Autodesk Inventor part; units mm, degrees
ref_plane "YZ Plane" through (0, 0, 0) normal (1, 0, 0) x (0, 1, 0)
ref_plane "XZ Plane" through (0, 0, 0) normal (0, 1, 0) x (-1, 0, 0)
ref_plane "XY Plane" through (0, 0, 0) normal (0, 0, 1) x (1, 0, 0)
sketch "Sketch1" plane through (0, 0, 0) normal (0, 1, 0) x (-1, 0, 0)
  line L0 (-1.27, 1.27) -> (1.27, 1.27)
  line L1 (1.27, 1.27) -> (1.27, -1.27)
  line L2 (1.27, -1.27) -> (-1.27, -1.27)
  line L3 (-1.27, -1.27) -> (-1.27, 1.27)
  line L4 (-1.27, 1.27) -> (1.27, -1.27) construction
  line L5 (1.27, 1.27) -> (-1.27, -1.27) construction
  point P0 (0, 0)
  dimension "d0" = 2.54
  dimension "d1" = 2.54
extrude "Extrusion1" add sketch "Sketch1" along normal blind 10
sketch "Sketch2" plane through (0, 10, 0) normal (0, 1, 0) x (1, 0, 0)
  circle A0 centre (0, 0) radius 0.375
  dimension "d4" = 0.75
extrude "Extrusion2" cut sketch "Sketch2" against normal blind 100
fillet "Fillet1" radius 0.5 4 edges at (-1.27, 5, 1.27) (1.27, 5, 1.27) (1.27, 5, -1.27) (-1.27, 5, -1.27)
properties part number "block"
Verification items for the finished model (mm, model axes). Round coordinates to 2 decimals unless told otherwise and drop trailing zeros. Order: outer loops, then holes, each group sorted by start corner. A loop starts at its lowest first (then second) coordinate and runs counter-clockwise, first axis right, second up. Notation, with made-up numbers: (80, 8.5) -> (90, 8.5) arc R27 ccw to (90, 33.5) -> close; hole circle Ø4 at (10.5, 57.25). An arc over 180 degrees is marked (long way). Put each result on its own line as item: value. Start each with the question number.
(1) Material ranges on line 1 along X through (y, z) = (4.5, 0) (3 decimals); line 2 along Z through (x, y) = (-0.9, 4), recorded low to high.
(2) Section check B-B (x = 0). Enter the section's corners in (y, z) (3 decimals), then the cut area to 3 significant figures.
(3) Depth check by flat-ended pin: pin 1 Ø1.5 at (y, z) = (1, 1) entering from -X. Enter the tip coordinate at first touch or a pass-through.
(4) Section check D-D (z = 0.95). Enter the section's corners in (x, y), then the cut area to 3 significant figures.
(5) Section check A-A (z = 0). Enter the section's corners in (x, y) (3 decimals), then the cut area to 3 significant figures.
(6) Section check C-C (y = 6). Enter the section's corners in (x, z) (3 decimals).
Completed:
1. line 1: x = -1.27 to -0.375, 0.375 to 1.27
1. line 2: z = -1.25 to 1.25
2. outline: (0, -1.27) -> (10, -1.27) -> (10, -0.375) -> (0, -0.375) -> close; (0, 0.375) -> (10, 0.375) -> (10, 1.27) -> (0, 1.27) -> close
2. area: 17.9 mm2
3. pin 1: stops at x = -1.27
4. outline: (-1.24, 0) -> (1.24, 0) -> (1.24, 10) -> (-1.24, 10) -> close
4. area: 24.7 mm2
5. outline: (-1.27, 0) -> (-0.375, 0) -> (-0.375, 10) -> (-1.27, 10) -> close; (0.375, 0) -> (1.27, 0) -> (1.27, 10) -> (0.375, 10) -> close
5. area: 17.9 mm2
6. outline: (-1.27, -0.77) arc R0.5 ccw to (-0.77, -1.27) -> (0.77, -1.27) arc R0.5 ccw to (1.27, -0.77) -> (1.27, 0.77) arc R0.5 ccw to (0.77, 1.27) -> (-0.77, 1.27) arc R0.5 ccw to (-1.27, 0.77) -> close; hole circle Ø0.75 at (0, 0)
